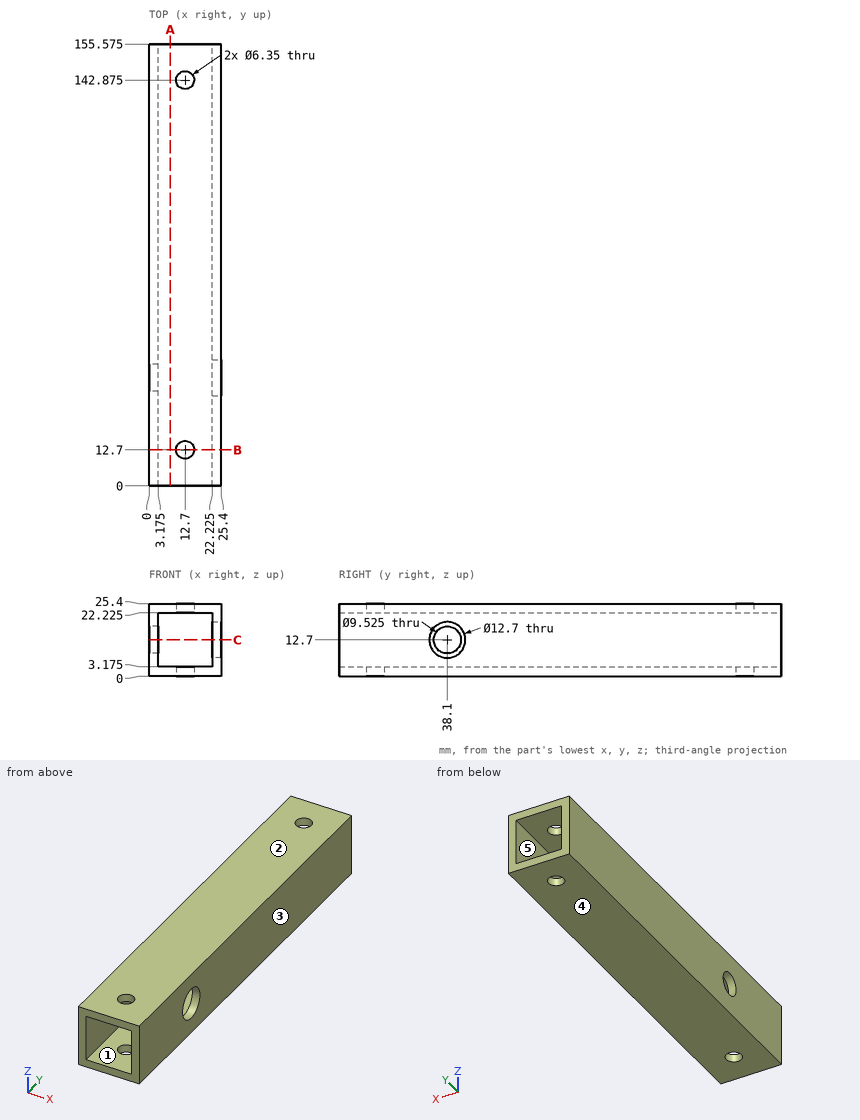
The drawing under review shows one solid part. Ordinate dimensions are in mm from its lowest x, y, z. A direction names the side the tool comes from. Give positions to 0.01 mm unless a question says otherwise; leave off trailing zeros. Order: outer loops, then holes, each group sorted by start corner. A loop starts at its lowest first (then second) coordinate and runs counter-clockwise, first axis right, second up. Notation, with made-up numbers: (-30.75, -27.75) -> (-3.75, -27.75) arc R18 ccw to (-3.75, -18.75) -> close; hole circle Ø6 at (-34.5, 80.5). An arc over 180 degrees is marked (long way). Write item = value, one per line. Start each with the question number.
(1) We need section A-A on x = 7.5. Write out the cut boundary in (y, z) (3 decimals).
(2) We need section B-B on y = 12.7. Write out the cut boundary in (x, z) (3 decimals).
(3) We need section C-C on z = 12.7. State how many separate pieces and enclosed holes the cut face has, plus the area to 3 significant figures.
(4) For pin 1 (8.5 mm diameter, centred on y = 38.1, z = 12.7, fed in from +X), flat-tipped, find the tip position at first contact; note if it passes through.
(5) For the marked faces 4 and 5, list the 3-axis set-ups (+Z, -Z, +X, -X, +Y, -Y) from which the entire face can be reached by the end or side of a thin tool; tool diameter is ignored.
(6) To check wall thickness, follow line 1 along Y through (x, z) = (12.7, 2.4) (3 decimals); line 2 along X through (y, z) = (75, 7.25) (3 decimals). State the ranges of each line that lie inside material, in increasing order.
(7) Mouldability with a two-part tool opening along X and no side actions: class the marked faces 1, 2 and 3 as +X half, -X half, draft (parallel to the pull), parting line (faces both ways), or undercut.
Numbers:
q1.outline = (0, 0) -> (155.575, 0) -> (155.575, 3.175) -> (0, 3.175) -> close; (0, 22.225) -> (155.575, 22.225) -> (155.575, 25.4) -> (0, 25.4) -> close
q2.outline = (0, 0) -> (9.525, 0) -> (9.525, 3.175) -> (3.175, 3.175) -> (3.175, 22.225) -> (9.525, 22.225) -> (9.525, 25.4) -> (0, 25.4) -> close; (15.875, 0) -> (25.4, 0) -> (25.4, 25.4) -> (15.875, 25.4) -> (15.875, 22.225) -> (22.225, 22.225) -> (22.225, 3.175) -> (15.875, 3.175) -> close
q3.separate_pieces = 4
q3.enclosed_holes = 0
q3.area = 917 mm^2
q4.pin_1 = through
q5.face_4 = -Z, +X, -X, +Y, -Y
q5.face_5 = +Y, -Y
q6.line_1 = 0 to 9.525, 15.875 to 139.7, 146.05 to 155.575
q6.line_2 = 0 to 3.175, 22.225 to 25.4
q7.face_1 = undercut
q7.face_2 = draft
q7.face_3 = +X half
